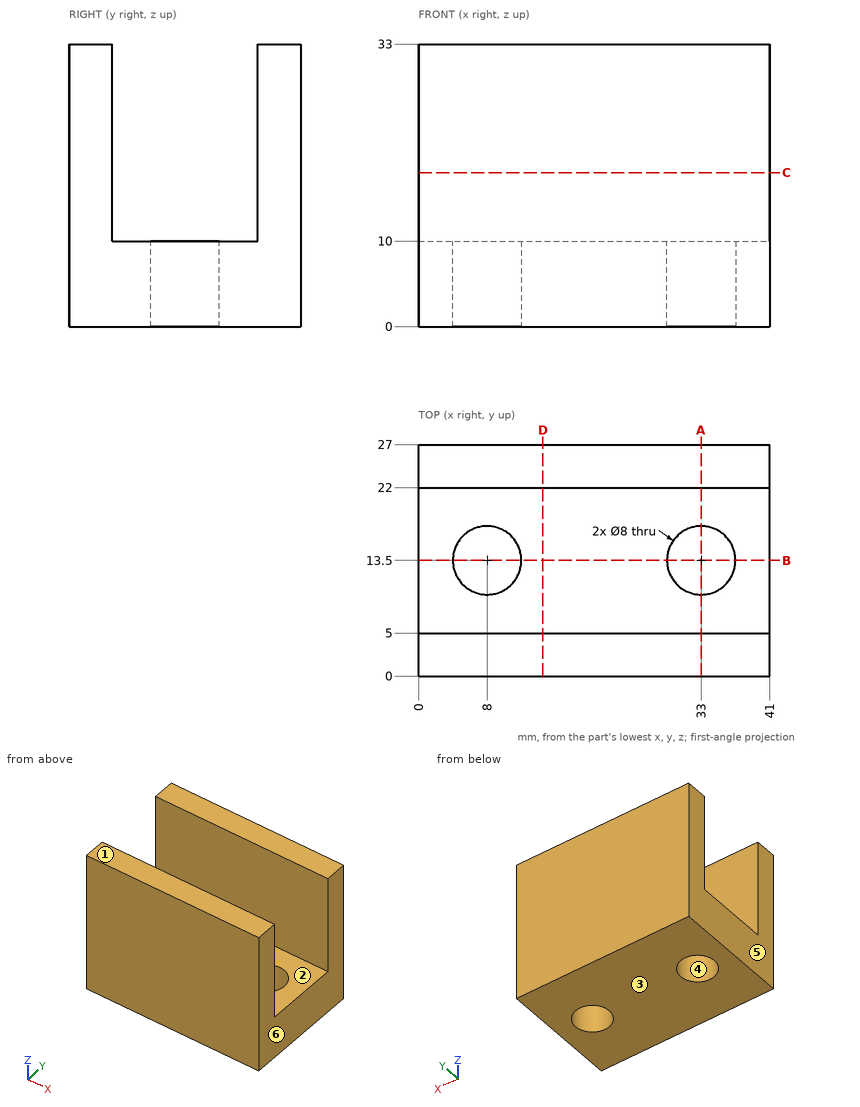
Verification items for this drawing (mm, ordinates from the low corner). A direction names the side the tool comes from. Round coordinates to 2 decimals unless told otherwise and drop trailing zeros. Loops run counter-clockwise (first coordinate to the right, second up) from the corner with the lowest first, then second, coordinate; pieces in that order, holes last. Notation, with made-up numbers: (67, 25) - (71, 25) arc R14 cw to (71, 43) - close; hole circle Ø9 at (28.5, 49). An arc over 180 degrees is marked (long way). Write item = value, one per line.
Q1. Sectioned sample at B-B on y = 13.5. Record the boundary of the cut face in (x, z), plus the area to 3 significant figures.
Here are the results:
outline = (0, 0) - (4, 0) - (4, 10) - (0, 10) - close; (12, 0) - (29, 0) - (29, 10) - (12, 10) - close; (37, 0) - (41, 0) - (41, 10) - (37, 10) - close
area = 250 mm^2
Q2. Tool access check on the marked faces 1 and 2. Record the directions out of +Z, -Z, +X, -X, +Y, -Y that give a thin tool (end or side, any length) a straight path to the whole face; none if there is none.
Here are the results:
face_1 = +Z, +X, -X, +Y, -Y
face_2 = +Z, +X, -X
Q3. Sectioned sample at A-A on x = 33. Record the boundary of the cut face in (y, z).
Here are the results:
outline = (0, 0) - (9.5, 0) - (9.5, 10) - (5, 10) - (5, 33) - (0, 33) - close; (17.5, 0) - (27, 0) - (27, 33) - (22, 33) - (22, 10) - (17.5, 10) - close
Q4. Sectioned sample at C-C on z = 18. Record the boundary of the cut face in (x, y).
Here are the results:
outline = (0, 0) - (41, 0) - (41, 5) - (0, 5) - close; (0, 22) - (41, 22) - (41, 27) - (0, 27) - close
Q5. Sectioned sample at D-D on x = 14.5. Record the boundary of the cut face in (y, z), plus the area to 3 significant figures.
Here are the results:
outline = (0, 0) - (27, 0) - (27, 33) - (22, 33) - (22, 10) - (5, 10) - (5, 33) - (0, 33) - close
area = 500 mm^2
Q6. Depth check by flat-ended pin: pin 1 (1 mm diameter, centred on x = 18, z = 28, fed in from -Y); pin 2 (3 mm diameter, centred on x = 15, y = 15.5, fed in from +Z); pin 3 (7 mm diameter, centred on x = 33, y = 13.5, fed in from -Z) (1 decimal). Enter the tip coordinate at first touch or a pass-through.
Here are the results:
pin_1 = 0
pin_2 = 10
pin_3 = through
Q7. Material ranges on L1, parallel to Y at x = 23.5, z = 31; L2, parallel to Y at x = 8, z = 3; L3, parallel to Z at x = 21, y = 18.25, recorded low to high.
Here are the results:
L1 = 0 to 5, 22 to 27
L2 = 0 to 9.5, 17.5 to 27
L3 = 0 to 10
Q8. Mould release check, pull along X, two halves, no side actions. Record for the marked faces 3, 4, 5 and 6: +X half, -X half, draft (parallel to the pull), parting line (faces both ways), or undercut.
Here are the results:
face_3 = draft
face_4 = undercut
face_5 = -X half
face_6 = +X half
